```python
from build123d import *

# Parameters (mm, degrees)
SKETCH1_W           = 69.025336674
SKETCH1_H           = 89.501461159
SKETCH1_W_2         = 62.929336674
SKETCH1_H_2         = 83.405461159
SKETCH1_W_3         = 10.637877579
SKETCH1_H_3         = 2.400289179
SKETCH1_W_4         = 10.76808562
SKETCH1_H_4         = 2.410116194
SKETCH1_W_5         = 10.845055727
SKETCH1_H_5         = 2.320385117
SKETCH1_W_6         = 8.61961261
SKETCH1_W_7         = 8.696582717
SKETCH1_W_8         = 7.233122671
SKETCH1_H_6         = 1.406184517
SKETCH1_W_9         = 7.693154637
SKETCH1_H_7         = 1.374601098
SKETCH1_W_10        = 4.85814416
SKETCH1_H_8         = 1.33271236
SKETCH1_W_11        = 5.120398278
SKETCH1_H_9         = 1.332092237
SKETCH1_W_12        = 6.797362186
SKETCH1_H_10        = 1.320409981
SKETCH1_W_13        = 10.954732913
SKETCH1_H_11        = 2.291459462
SKETCH1_W_14        = 13.940499857
SKETCH1_H_12        = 1.597280353
SKETCH1_W_15        = 11.193978309
SKETCH1_W_16        = 8.509935424
SKETCH1_W_17        = 8.826790758
SKETCH1_H_13        = 2.316503995
SKETCH1_W_18        = 8.117773256
SKETCH1_H_14        = 1.391011178
SKETCH1_W_19        = 7.14925004
SKETCH1_W_20        = 4.435758543
BOSS_EXTRUDE1_DEPTH = 2.54


with BuildPart() as part:
    # Sketch1 → Boss-Extrude1 (new body)
    # profile 1 of 20: a face of its own
    with BuildSketch(Plane.XY):
        with Locations((-59.696453639, 17.511447337)):
            Rectangle(SKETCH1_W, SKETCH1_H)
        with Locations((-59.696453639, 17.511447337)):
            Rectangle(SKETCH1_W_2, SKETCH1_H_2, mode=Mode.SUBTRACT)
    # profile 2 of 20: a face of its own
    with BuildSketch(Plane.XY):
        with Locations((-85.842183186, 53.603021221)):
            Rectangle(SKETCH1_W_3, SKETCH1_H_3)
    # profile 3 of 20: a face of its own
    with BuildSketch(Plane.XY):
        with Locations((-85.777079166, 35.533767551)):
            Rectangle(SKETCH1_W_4, SKETCH1_H_4)
    # profile 4 of 20: a face of its own
    with BuildSketch(Plane.XY):
        with Locations((-85.738594113, 17.477618848)):
            Rectangle(SKETCH1_W_5, SKETCH1_H_5)
    # profile 5 of 20: a face of its own
    with BuildSketch(Plane.XY):
        with Locations((-64.006259944, 17.477618848)):
            Rectangle(SKETCH1_W_6, SKETCH1_H_5)
    # profile 6 of 20: a face of its own
    with BuildSketch(Plane.XY):
        with Locations((-64.044744998, 35.533767551)):
            Rectangle(SKETCH1_W_7, SKETCH1_H_4)
    # profile 7 of 20: a face of its own
    with BuildSketch(Plane.XY):
        Polygon((-56.648453639, 59.214177916), (-59.696453639, 59.214177916), (-59.696453639, 54.719380626), (-59.696453639, 52.402876631), (-59.696453639, 36.738825648), (-59.696453639, 34.328709454), (-59.696453639, 18.637811406), (-59.696453639, 16.317426289), (-59.696453639, 0.495724739), (-59.696453639, -1.795734723), (-59.696453639, -15.430210162), (-59.696453639, -17.027490515), (-59.696453639, -24.191283243), (-56.648453639, -24.191283243), (-56.648453639, -16.118247947), (-56.648453639, -14.797837966), (-56.648453639, 6.731660618), (-56.648453639, 8.064372978), (-56.648453639, 29.090462814), (-56.648453639, 30.496647331), (-56.648453639, 49.145727963), (-56.648453639, 50.536739141), align=None)
    # profile 8 of 20: a face of its own
    with BuildSketch(Plane.XY):
        with Locations((-53.031892304, 29.793555073)):
            Rectangle(SKETCH1_W_8, SKETCH1_H_6)
    # profile 9 of 20: a face of its own
    with BuildSketch(Plane.XY):
        with Locations((-32.078362621, 29.946844808)):
            Rectangle(SKETCH1_W_9, SKETCH1_H_7)
    # profile 10 of 20: a face of its own
    with BuildSketch(Plane.XY):
        with Locations((-30.660857382, 7.398016798)):
            Rectangle(SKETCH1_W_10, SKETCH1_H_8)
    # profile 11 of 20: a face of its own
    with BuildSketch(Plane.XY):
        with Locations((-30.791984441, -14.131791848)):
            Rectangle(SKETCH1_W_11, SKETCH1_H_9)
    # profile 12 of 20: a face of its own
    with BuildSketch(Plane.XY):
        with Locations((-53.249772546, -15.458042957)):
            Rectangle(SKETCH1_W_12, SKETCH1_H_10)
    # profile 13 of 20: a face of its own
    with BuildSketch(Plane.XY):
        with Locations((-85.68375552, -0.650004992)):
            Rectangle(SKETCH1_W_13, SKETCH1_H_11)
    # profile 14 of 20: a face of its own
    with BuildSketch(Plane.XY):
        with Locations((-84.190872047, -16.228850339)):
            Rectangle(SKETCH1_W_14, SKETCH1_H_12)
    # profile 15 of 20: a face of its own
    with BuildSketch(Plane.XY):
        with Locations((-65.293442794, -16.228850339)):
            Rectangle(SKETCH1_W_15, SKETCH1_H_12)
    # profile 16 of 20: a face of its own
    with BuildSketch(Plane.XY):
        with Locations((-63.951421351, -0.650004992)):
            Rectangle(SKETCH1_W_16, SKETCH1_H_11)
    # profile 17 of 20: a face of its own
    with BuildSketch(Plane.XY):
        with Locations((-64.109849018, 53.561128629)):
            Rectangle(SKETCH1_W_17, SKETCH1_H_13)
    # profile 18 of 20: a face of its own
    with BuildSketch(Plane.XY):
        with Locations((-32.29067193, 49.841233552)):
            Rectangle(SKETCH1_W_18, SKETCH1_H_14)
    # profile 19 of 20: a face of its own
    with BuildSketch(Plane.XY):
        with Locations((-53.073828619, 49.841233552)):
            Rectangle(SKETCH1_W_19, SKETCH1_H_14)
    # profile 20 of 20: a face of its own
    with BuildSketch(Plane.XY):
        with Locations((-54.430574368, 7.398016798)):
            Rectangle(SKETCH1_W_20, SKETCH1_H_8)
    extrude(amount=BOSS_EXTRUDE1_DEPTH)


solid = part.part
```
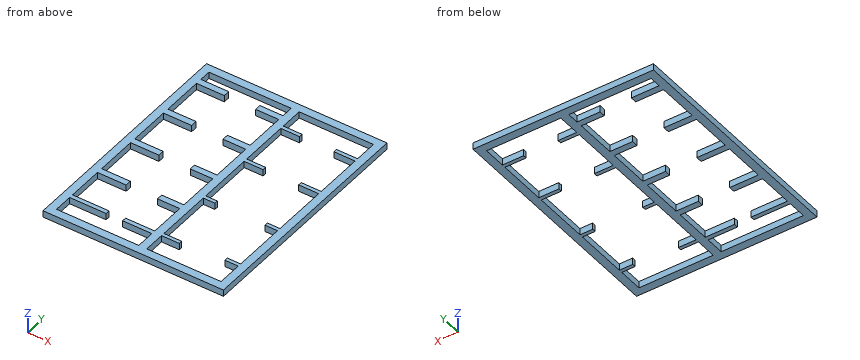
Design review of the part built by this model. Coordinates are the model's own, in mm. Give positions to 0.01 mm unless a question says otherwise; leave off trailing zeros. Loops run counter-clockwise (first coordinate to the right, second up) from the corner with the lowest first, then second, coordinate; pieces in that order, holes last. Notation, with made-up numbers: (40, 28.5) -> (90, 28.5) arc R17 ccw to (90, 44.5) -> close; hole circle Ø1 at (73, 53). An arc over 180 degrees is marked (long way). One line per item, written item: value.
Q1. For pin 1 Ø8 at (x, y) = (-66, 29) entering from +Z, flat-tipped, find the tip position at first contact; note if it passes through.
Numbers:
pin 1: passes through
Q2. We need section D-D on x = -29.5. Give the boundary of the cut face in (y, z), and give its area (3 significant figures).
Numbers:
outline: (-27.24, 0) -> (-24.19, 0) -> (-24.19, 2.54) -> (-27.24, 2.54) -> close; (-14.8, 0) -> (-13.47, 0) -> (-13.47, 2.54) -> (-14.8, 2.54) -> close; (6.73, 0) -> (8.06, 0) -> (8.06, 2.54) -> (6.73, 2.54) -> close; (29.26, 0) -> (30.63, 0) -> (30.63, 2.54) -> (29.26, 2.54) -> close; (49.15, 0) -> (50.54, 0) -> (50.54, 2.54) -> (49.15, 2.54) -> close; (59.21, 0) -> (62.26, 0) -> (62.26, 2.54) -> (59.21, 2.54) -> close
area: 29.3 mm^2
Q3. We need section B-B on y = 47. Give the boundary of the cut face in (x, z).
Numbers:
outline: (-94.21, 0) -> (-91.16, 0) -> (-91.16, 2.54) -> (-94.21, 2.54) -> close; (-59.7, 0) -> (-56.65, 0) -> (-56.65, 2.54) -> (-59.7, 2.54) -> close; (-28.23, 0) -> (-25.18, 0) -> (-25.18, 2.54) -> (-28.23, 2.54) -> close
Q4. We need section A-A on x = -76. Give the boundary of the cut face in (y, z).
Numbers:
outline: (-27.24, 0) -> (-24.19, 0) -> (-24.19, 2.54) -> (-27.24, 2.54) -> close; (59.21, 0) -> (62.26, 0) -> (62.26, 2.54) -> (59.21, 2.54) -> close
Q5. For L1, parallel to Y at x = -51.5, z = 1.65; L2, parallel to Y at x = -70, z = 1.1; L3, parallel to X at y = 18, z = 0.8, list the stretches that pass through material, from the lowest coordinate up.
Numbers:
L1: y = -27.24 to -24.19, -16.12 to -14.8, 29.09 to 30.5, 49.15 to 50.54, 59.21 to 62.26
L2: y = -27.24 to -24.19, -17.03 to -15.43, 59.21 to 62.26
L3: x = -94.21 to -80.32, -68.32 to -56.65, -28.23 to -25.18
Q6. We need section C-C on x = -63.5. Give the boundary of the cut face in (y, z), and give its area (3 significant figures).
Numbers:
outline: (-27.24, 0) -> (-24.19, 0) -> (-24.19, 2.54) -> (-27.24, 2.54) -> close; (-17.03, 0) -> (-15.43, 0) -> (-15.43, 2.54) -> (-17.03, 2.54) -> close; (-1.8, 0) -> (0.5, 0) -> (0.5, 2.54) -> (-1.8, 2.54) -> close; (16.32, 0) -> (18.64, 0) -> (18.64, 2.54) -> (16.32, 2.54) -> close; (34.33, 0) -> (36.74, 0) -> (36.74, 2.54) -> (34.33, 2.54) -> close; (52.4, 0) -> (54.72, 0) -> (54.72, 2.54) -> (52.4, 2.54) -> close; (59.21, 0) -> (62.26, 0) -> (62.26, 2.54) -> (59.21, 2.54) -> close
area: 43.3 mm^2
